The listing builds one solid part. Answer for the finished solid, in the listing's coordinates (mm). Face numbers are marked on the shaded views. A direction names the side the tool comes from. Coordinates: 2 decimals unless noted, no trailing zeros. Loops run counter-clockwise (first coordinate to the right, second up) from the corner with the lowest first, then second, coordinate; pieces in that order, holes last. Notation, with made-up numbers: (-26, -12.75) -> (-3, -12.75) arc R30 ccw to (-3, 18.25) -> close; hole circle Ø2 at (-31.75, 58). An arc over 180 degrees is marked (long way). Answer in a Markdown table with one row per item.
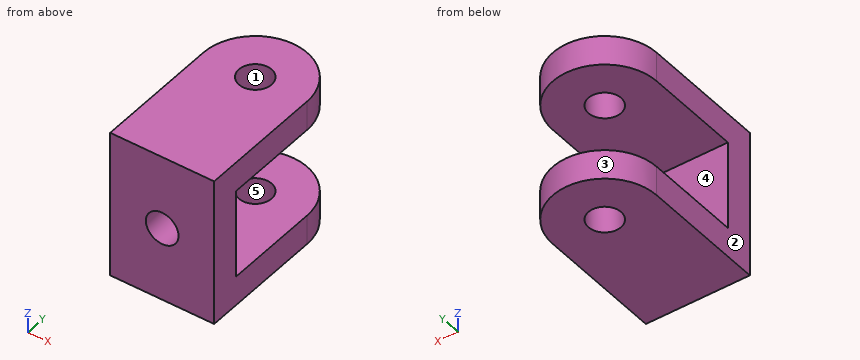
```python
from build123d import *

# Parameters (mm, degrees)
SKETCH_1_W          = 7
SKETCH_1_H          = 10
EXTRUDE_1_DEPTH     = 2
SKETCH_2_W          = 7
SKETCH_2_H          = 2
EXTRUDE_2_DEPTH     = 10
FILLET_1_RADIUS     = 3.5
FILLET_1_LENGTH     = 2
FILLET_2_RADIUS     = 3.5
FILLET_2_LENGTH     = 2
SKETCH_3_R          = 1.1
CUT_EXTRUDE_1_DEPTH = 25
SKETCH_4_R          = 1.1
CUT_EXTRUDE_2_DEPTH = 25


with BuildPart() as part:
    # 草图1 → 凸台-拉伸1 (new body)
    with BuildSketch(Plane(origin=(0, 0, 0), x_dir=(1, 0, 0), z_dir=(0, 1, 0))):
        Rectangle(SKETCH_1_W, SKETCH_1_H)
    extrude(amount=EXTRUDE_1_DEPTH)

    # 草图2 → 凸台-拉伸2 (add)
    with BuildSketch(Plane(origin=(0, 2, 0), x_dir=(1, 0, 0), z_dir=(0, 1, 0))):
        with Locations((0, -4)):
            Rectangle(SKETCH_2_W, SKETCH_2_H)
        with Locations((0, 4)):
            Rectangle(SKETCH_2_W, SKETCH_2_H)
    extrude(amount=EXTRUDE_2_DEPTH)

    # 圆角1: full round fillet: the end face becomes a half cylinder, R = half its width
    fillet_1_face = Plane((0, 12, 4), x_dir=(0, 0, 1), z_dir=(0, 1, 0))  # on the end face: x along it, z out of the body
    fillet_1_slab = fillet_1_face.offset(-FILLET_1_RADIUS / 2) * Box(FILLET_1_LENGTH, 2 * FILLET_1_RADIUS, FILLET_1_RADIUS, mode=Mode.PRIVATE)  # the body's end, R deep
    fillet_1_round = Plane((0, 8.5, 4), x_dir=(0, 1, 0), z_dir=(0, 0, 1)) * Cylinder(FILLET_1_RADIUS, FILLET_1_LENGTH, mode=Mode.PRIVATE)  # its axis R under the face
    add(fillet_1_slab - fillet_1_round, mode=Mode.SUBTRACT)

    # 圆角2: full round fillet: the end face becomes a half cylinder, R = half its width
    fillet_2_face = Plane((0, 12, -4), x_dir=(0, 0, 1), z_dir=(0, 1, 0))  # on the end face: x along it, z out of the body
    fillet_2_slab = fillet_2_face.offset(-FILLET_2_RADIUS / 2) * Box(FILLET_2_LENGTH, 2 * FILLET_2_RADIUS, FILLET_2_RADIUS, mode=Mode.PRIVATE)  # the body's end, R deep
    fillet_2_round = Plane((0, 8.5, -4), x_dir=(0, 1, 0), z_dir=(0, 0, 1)) * Cylinder(FILLET_2_RADIUS, FILLET_2_LENGTH, mode=Mode.PRIVATE)  # its axis R under the face
    add(fillet_2_slab - fillet_2_round, mode=Mode.SUBTRACT)

    # 草图3 → 切除-拉伸1 (cut)
    with BuildSketch(Plane(origin=(0, 0, -5), x_dir=(-1, 0, 0), z_dir=(0, 0, -1))):
        with Locations((0, 8.5)):
            Circle(SKETCH_3_R)
    extrude(amount=-CUT_EXTRUDE_1_DEPTH, mode=Mode.SUBTRACT)

    # 草图4 → 切除-拉伸2 (cut)
    with BuildSketch(Plane(origin=(0, 2, 0), x_dir=(1, 0, 0), z_dir=(0, 1, 0))):
        with Locations(Location((0, 0, 0), (0, 0, 270))):
            Circle(SKETCH_4_R)
    extrude(amount=-CUT_EXTRUDE_2_DEPTH, mode=Mode.SUBTRACT)


solid = part.part
```
Item 1: Find the intervals of material crossed by probe 1 along Z at (x, y) = (-1.5, 6); probe 2 along Y at (x, z) = (0, -4.1); probe 3 along X at (y, z) = (1.35, 0), in increasing order.
Findings below:
| item | result |
|---|---|
| probe 1 | z = -5 to -3, 3 to 5 |
| probe 2 | y = 0 to 7.4, 9.6 to 12 |
| probe 3 | x = -3.5 to -1.1, 1.1 to 3.5 |
Item 2: Flat-ended cylindrical pins translate along their axes: pin 1 Ø1 at (x, y) = (1, 8.5) entering from -Z; pin 2 Ø1.5 at (x, z) = (1, -4) entering from +Y; pin 3 Ø3 at (x, z) = (-1.5, 0) entering from +Y; pin 4 Ø1.5 at (y, z) = (8.5, 2) entering from +X. Find the tip coordinate at first contact, or state that the pin passes through.
Findings below:
| item | result |
|---|---|
| pin 1 | stops at z = -5 |
| pin 2 | stops at y = 11.99 |
| pin 3 | stops at y = 2 |
| pin 4 | passes through |
Item 3: A cutting plane is placed at D-D, the plane x = -2.5. Determine the outline of the cut face in (y, z), plus the area to 3 significant figures.
Findings below:
| item | result |
|---|---|
| outline | (0, -5) -> (10.95, -5) -> (10.95, -3) -> (2, -3) -> (2, 3) -> (10.95, 3) -> (10.95, 5) -> (0, 5) -> close |
| area | 55.8 mm2 |
Item 4: A tool of negligible diameter and unlimited length cuts with its end or side. For the marked faces 4 and 5, from which of +Z, -Z, +X, -X, +Y, -Y can it reach the whole face along a straight path? Write none if from no direction.
Findings below:
| item | result |
|---|---|
| face 4 | +X, -X, +Y |
| face 5 | +Z, -Z |
Item 5: Determine the mould class of the marked faces 1, 2 and 3 for opening direction Y: +Y half, -Y half, draft (parallel to the pull), parting line (faces both ways), or undercut.
Findings below:
| item | result |
|---|---|
| face 1 | undercut |
| face 2 | draft |
| face 3 | +Y half |
Item 6: A cutting plane is placed at B-B, the plane y = 4.5. Determine the outline of the cut face in (x, z), plus the area to 3 significant figures.
Findings below:
| item | result |
|---|---|
| outline | (-3.5, -5) -> (3.5, -5) -> (3.5, -3) -> (-3.5, -3) -> close; (-3.5, 3) -> (3.5, 3) -> (3.5, 5) -> (-3.5, 5) -> close |
| area | 28.0 mm2 |
Item 7: A cutting plane is placed at A-A, the plane x = 0. Determine the outline of the cut face in (y, z), plus the area to 3 significant figures.
Findings below:
| item | result |
|---|---|
| outline | (0, -5) -> (7.4, -5) -> (7.4, -3) -> (2, -3) -> (2, -1.1) -> (0, -1.1) -> close; (0, 1.1) -> (2, 1.1) -> (2, 3) -> (7.4, 3) -> (7.4, 5) -> (0, 5) -> close; (9.6, -5) -> (12, -5) -> (12, -3) -> (9.6, -3) -> close; (9.6, 3) -> (12, 3) -> (12, 5) -> (9.6, 5) -> close |
| area | 46.8 mm2 |
Item 8: A cutting plane is placed at C-C, the plane z = 0. Determine the outline of the cut face in (x, y).
Findings below:
| item | result |
|---|---|
| outline | (-3.5, 0) -> (-1.1, 0) -> (-1.1, 2) -> (-3.5, 2) -> close; (1.1, 0) -> (3.5, 0) -> (3.5, 2) -> (1.1, 2) -> close |
